from build123d import *

# Parameters (mm, degrees)
F0_W     = 50
F0_H     = 13
F0_R     = 2
F0_R_2   = 4
F1_DEPTH = 3
F2_R     = 5


with BuildPart() as f1:
    # F0 (on Top) → F1 (new body)
    with BuildSketch(Plane.XY):
        with Locations((0, 0.5)):
            Rectangle(F0_W, F0_H)
        with Locations((0, -3)):
            Circle(F0_R, mode=Mode.SUBTRACT)
        with Locations((-14.25, 2)):
            Circle(F0_R_2, mode=Mode.SUBTRACT)
        with Locations((14.25, 2)):
            Circle(F0_R_2, mode=Mode.SUBTRACT)
    extrude(amount=F1_DEPTH)

    # F2
    f2_edges = [f1.edges().sort_by_distance(p)[0] for p in [
        (-25, 7, 1.5),
        (-25, -6, 1.5),
        (25, -6, 1.5),
        (25, 7, 1.5),
    ]]
    fillet(f2_edges, radius=F2_R)


solid = f1.part
Check sheet for the modelled part. Datum: model origin and axes. Units: mm. Round coordinates to 2 decimals unless told otherwise and drop trailing zeros. Write each loop counter-clockwise with the first axis right and the second up, starting at its lowest first coordinate (ties: lowest second). Pieces come first, ordered by that corner, then holes. Notation, with made-up numbers: (46.5, 11.5) - (99.5, 11.5) arc R7 ccw to (99.5, 18.5) - close; hole circle Ø11 at (-32, 39.5). An arc over 180 degrees is marked (long way). Return JSON: item names as keys, results as strings.
Q1. Draft check along X on faces 1 (the cylindrical face through (0, -5, 1)), 2 (the flat face through (0, 7, 1)), 3 (the cylindrical face through (10.254, 2.176, 1.479)), 4 (the cylindrical face through (-24, -4, 2)). Enter one of: released by +X, released by -X, zero draft, split by the parting line, or undercut.
Returned:
{"face 1": "undercut", "face 2": "zero draft", "face 3": "undercut", "face 4": "released by -X"}
Q2. Scan lines: L1, parallel to Y at x = -14.25, z = 1.45; L2, parallel to X at y = -1.5, z = 0.3; L3, parallel to Y at x = 0, z = 2.1. Record each from-to range of solid material in increasing order. Write a range as from..to.
Returned:
{"L1": "y = -6..-2, 6..7", "L2": "x = -24.97..-16.19, -12.31..-1.32, 1.32..12.31, 16.19..24.97", "L3": "y = -6..-5, -1..7"}
Q3. Cross-section at C-C (y = -3). Record the boundary of the cut face in (x, z).
Returned:
{"outline": "(-24.58, 0) - (-2, 0) - (-2, 3) - (-24.58, 3) - close; (2, 0) - (24.58, 0) - (24.58, 3) - (2, 3) - close"}
Q4. Cross-section at D-D (y = 0). Record the boundary of the cut face in (x, z).
Returned:
{"outline": "(-25, 0) - (-17.71, 0) - (-17.71, 3) - (-25, 3) - close; (-10.79, 0) - (10.79, 0) - (10.79, 3) - (-10.79, 3) - close; (17.71, 0) - (25, 0) - (25, 3) - (17.71, 3) - close"}
Q5. Cross-section at B-B (z = 0.7). Record the boundary of the cut face in (x, y), then the cut area to 3 significant figures.
Returned:
{"outline": "(-25, -1) arc R5 ccw to (-20, -6) - (20, -6) arc R5 ccw to (25, -1) - (25, 2) arc R5 ccw to (20, 7) - (-20, 7) arc R5 ccw to (-25, 2) - close; hole circle Ø8 at (-14.25, 2); hole circle Ø4 at (0, -3); hole circle Ø8 at (14.25, 2)", "area": "515 mm²"}
Q6. Cross-section at A-A (x = -14.25). Record the boundary of the cut face in (y, z).
Returned:
{"outline": "(-6, 0) - (-2, 0) - (-2, 3) - (-6, 3) - close; (6, 0) - (7, 0) - (7, 3) - (6, 3) - close"}
Q7. Depth check by flat-ended pin: P1, Ø7, axis at x = 14.25, y = 2, coming from the -Z side; P2, Ø4.5, axis at x = 0, y = -3, coming from the +Z side. Enter the tip coordinate at first touch or a pass-through.
Returned:
{"P1": "passes through", "P2": "stops at z = 3"}
